from build123d import *

# Parameters (mm, degrees)
BOSS_EXTRUDE1_DEPTH = 3
SKETCH2_W           = 5
SKETCH2_H           = 100
BOSS_EXTRUDE2_DEPTH = 3
SKETCH3_R           = 2.25
CUT_EXTRUDE1_DEPTH  = 3


with BuildPart() as part:
    # Sketch1 → Boss-Extrude1 (new body)
    with BuildSketch(Plane.XY):
        Polygon((-15.25, 50), (-15.25, 35), (-12.25, 35), (-12.25, 25), (-15.25, 25), (-15.25, -25), (-12.25, -25), (-12.25, -35), (-15.25, -35), (-15.25, -50), (-5, -50), (-5, -47), (5, -47), (5, -50), (15.25, -50), (15.25, 50), (5, 50), (5, 47), (-5, 47), (-5, 50), align=None)
    extrude(amount=BOSS_EXTRUDE1_DEPTH)

    # Sketch2 → Boss-Extrude2 (add)
    with BuildSketch(Plane.XY):
        with Locations((17.75, 0)):
            Rectangle(SKETCH2_W, SKETCH2_H)
    extrude(amount=BOSS_EXTRUDE2_DEPTH)

    # Sketch3 → Cut-Extrude1 (cut)
    with BuildSketch(Plane.XY.offset(3)):
        with Locations((15.25, 43.5)):
            Circle(SKETCH3_R)
    extrude(amount=-CUT_EXTRUDE1_DEPTH, mode=Mode.SUBTRACT)


solid = part.part
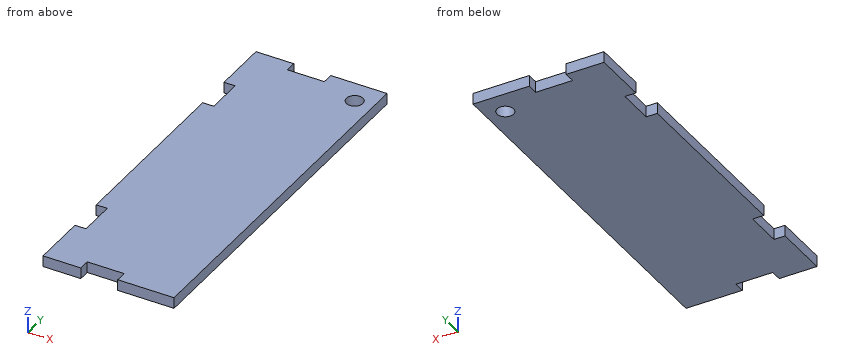
The listing builds one solid part. Answer for the finished solid, in the listing's coordinates (mm). Round coordinates to 2 decimals unless told otherwise and drop trailing zeros. Write each loop counter-clockwise with the first axis right and the second up, starting at its lowest first coordinate (ties: lowest second). Pieces come first, ordered by that corner, then holes. Notation, with made-up numbers: M 11,-10 L 58,-10 A11 cw 58,8 Z; hole C -32,4.5 d8. An arc over 180 degrees is marked long. Write each question's results on one line, items separated by ' | '. Start each with the question number.
(1) The part is cut by section A-A, the plane y = 43.5. Write down the section's boundary in (x, z).
(2) Find the intervals of material crossed by line 1 (Y direction, x = 15.25, z = 1.2); line 2 (X direction, y = -33.5, z = 0.5); line 3 (Y direction, x = -1, z = 2), in increasing order.
(3) The part is cut by section B-B, the plane x = 15.25. Write down the section's boundary in (y, z), and give its area (4 significant figures).
(4) The part is cut by section C-C, the plane z = 0.75. Write down the section's boundary in (x, y), and give its area (3 significant figures).
(5) The part is cut by section D-D, the plane y = -28. Write down the section's boundary in (x, z).
(6) Each of these flat-tipped pins is pushed along its axis until it touches: P1, Ø0.9, axis at y = -28.5, z = 2, coming from the -X side; P2, Ø0.9, axis at x = 1, z = 1.5, coming from the -Y side; P3, Ø0.9, axis at x = 2, z = 1, coming from the +Y side. Where does it stop, or does it pass through?
Worked answers:
1) outline: M -15.25,0 L 13,0 L 13,3 L -15.25,3 Z; M 17.5,0 L 20.25,0 L 20.25,3 L 17.5,3 Z
2) line 1: y = -50 to 41.25, 45.75 to 50 | line 2: x = -12.25 to 20.25 | line 3: y = -47 to 47
3) outline: M -50,0 L 41.25,0 L 41.25,3 L -50,3 Z; M 45.75,0 L 50,0 L 50,3 L 45.75,3 Z | area: 286.5 mm²
4) outline: M -15.25,-50 L -5,-50 L -5,-47 L 5,-47 L 5,-50 L 20.25,-50 L 20.25,50 L 5,50 L 5,47 L -5,47 L -5,50 L -15.25,50 L -15.25,35 L -12.25,35 L -12.25,25 L -15.25,25 L -15.25,-25 L -12.25,-25 L -12.25,-35 L -15.25,-35 Z; hole C 15.25,43.5 d4.5 | area: 3,410 mm²
5) outline: M -12.25,0 L 20.25,0 L 20.25,3 L -12.25,3 Z
6) P1: stops at x = -12.25 | P2: stops at y = -47 | P3: stops at y = 47
